```python
from build123d import *

# Parameters (mm, degrees)
SKETCH_1_R      = 1.45
EXTRUDE_1_DEPTH = 2
FILLET_1_R      = 5


with BuildPart() as part:
    # 草图1 → 凸台-拉伸1 (new body)
    with BuildSketch(Plane(origin=(0, 0, 0), x_dir=(1, 0, 0), z_dir=(0, 1, 0))):
        Polygon((651.168451136, -32.371101997), (650.079202112, -47.331500941), (680, -49.50999899), (681.089249024, -34.549600046), align=None)
        with Locations(Location((655.610626272, -40.214384477, 0), (0, 0, 270))):
            Circle(SKETCH_1_R, mode=Mode.SUBTRACT)
        with Locations(Location((675.557824864, -41.66671651, 0), (0, 0, 270))):
            Circle(SKETCH_1_R, mode=Mode.SUBTRACT)
    extrude(amount=EXTRUDE_1_DEPTH)

    # 圆角1
    fillet_1_edges = [part.edges().sort_by_distance(p)[0] for p in [
        (680, 1, 49.50999899),
        (650.079202112, 1, 47.331500941),
        (651.168451136, 1, 32.371101997),
        (681.089249024, 1, 34.549600046),
    ]]
    fillet(fillet_1_edges, radius=FILLET_1_R)


solid = part.part
```
Source: CAD feature listing. Evaluate the final solid. Frame: model axes, mm. Round coordinates to 2 decimals unless told otherwise and drop trailing zeros. Write each loop counter-clockwise with the first axis right and the second up, starting at its lowest first coordinate (ties: lowest second). Pieces come first, ordered by that corner, then holes. Notation, with made-up numbers: M 19,12.25 L 66,12.25 A16 cw 66,33.25 Z; hole C 4.5,-8 d1. An arc over 180 degrees is marked long. Answer as a JSON object with one key per item and string values. Group by question number.
(1) Section query A-A on z = 42. Output: boundary loops of the cut face in (x, y).
(2) Section query D-D on z = 36.5. Output: boundary loops of the cut face in (x, y).
(3) Mould query, pull axis Z, two halves, no side actions, for faces 1 (the flat face through (664.9, 0.99, 48.41)), 2 (the flat face through (666.27, 0.99, 33.47)), 3 (the cylindrical face through (677, 1, 41.5)), 4 (the flat face through (665, 2, 41)). Classes: +Z half, -Z half, draft (parallel to the pull), parting line (faces both ways), or undercut.
(4) Ray query, line 1 (Z direction, x = 655, y = 1.8); line 2 (Z direction, x = 654.5, y = 0.2); line 3 (X direction, y = 1, z = 42). Return the intervals inside material, ascending. Write a range as [from, to].
(5) Section query B-B on y = 0.6. Output: boundary loops of the cut face in (x, z).
(6) Section query C-C on x = 670.5. Output: boundary loops of the cut face in (y, z).
(7) First-contact query: pin 1 (8 mm diameter, centred on x = 655.5, z = 35.5, fed in from -Y). Flat tip, straight axial feed; report the tip coordinate or a pass-through.
Computed values:
{
 "1": {"outline": "M 650.47,0 L 674.15,0 L 674.15,2 L 650.47,2 Z; M 676.97,0 L 680.55,0 L 680.55,2 L 676.97,2 Z"},
 "2": {"outline": "M 650.94,0 L 679.96,0 L 679.96,2 L 650.94,2 Z"},
 "3": {"face 1": "+Z half", "face 2": "-Z half", "face 3": "undercut", "face 4": "draft"},
 "4": {"line 1": "[32.78, 38.9], [41.53, 47.69]", "line 2": "[32.89, 39.28], [41.15, 47.62]", "line 3": "[650.47, 674.15], [676.97, 680.55]"},
 "5": {"outline": "M 650.44,42.34 L 650.81,37.36 A5 ccw 656.16,32.73 L 676.1,34.19 A5 ccw 680.73,39.54 L 680.36,44.52 A5 ccw 675.01,49.15 L 655.07,47.69 A5 ccw Z; hole C 655.61,40.21 d2.9; hole C 675.56,41.67 d2.9"},
 "6": {"outline": "M 0,33.78 L 2,33.78 L 2,48.82 L 0,48.82 Z"},
 "7": {"pin 1": "y = 0"}
}
